```python
from build123d import *

# Parameters (mm, degrees)
SKETCH2_R          = 9.75
CUT_EXTRUDE1_DEPTH = 92.158049562


with BuildPart() as part:
    # Sketch1 → Revolve1 (revolve)
    with BuildSketch(Plane.XY, mode=Mode.PRIVATE) as revolve1_sk:
        Polygon((-17.25, 0), (-21.459646018, 0), (-23.940788684, 5.845205819), (-27.718503352, 5.845205819), (-30.199646018, 0), (-35, 0), (-35, 6.35), (-62.5, 6.35), (-62.5, 22.3), (-27, 22.3), (-27, 25), (-17.25, 25), align=None)
    revolve(revolve1_sk.sketch.rotate(Axis((0, 0, 0), (0, 1, 0)), 270), axis=Axis((0, 0, 0), (0, 1, 0)))

    # Sketch2 → Cut-Extrude1 (cut, through all)
    with BuildSketch(Plane(origin=(0, 22.3, 0), x_dir=(1, 0, 0), z_dir=(0, 1, 0))):
        with Locations(Location((-44.45, 0, 0), (0, 0, 270))):
            Circle(SKETCH2_R)
        with Locations(Location((0, 44.45, 0), (0, 0, 270))):
            Circle(SKETCH2_R)
        with Locations(Location((44.45, 0, 0), (0, 0, 270))):
            Circle(SKETCH2_R)
        with Locations(Location((0, -44.45, 0), (0, 0, 270))):
            Circle(SKETCH2_R)
    extrude(amount=-CUT_EXTRUDE1_DEPTH, mode=Mode.SUBTRACT)


solid = part.part
```
Work out the finished part from the listing and answer in its coordinate system (mm). A direction names the side the tool comes from. Give positions to 0.01 mm unless a question says otherwise; leave off trailing zeros. Order: outer loops, then holes, each group sorted by start corner. A loop starts at its lowest first (then second) coordinate and runs counter-clockwise, first axis right, second up. Notation, with made-up numbers: (63, 56.25) - (101, 56.25) arc R22 cw to (101, 63.25) - close; hole circle Ø4 at (88, -4). An arc over 180 degrees is marked (long way). One line per item, written item: value. Start each with the question number.
1. Section D-D, the plane z = -47 is taken. Write down the section's boundary in (x, y).
2. Section B-B, the plane z = 0 is taken. Write down the section's boundary in (x, y).
3. Which of the six approach directions +Z, -Z, +X, -X, +Y, -Y give full straight-line access (tool end or side, diameter ignored) to faces 1 (the face through (-24.999, 3.219, 24.496)), 2 (the face through (26.36, 23.67, 5.85)), 3 (the face through (12, 5.845, -21))?
4. Section C-C, the plane y = 11.25 is taken. Write down the section's boundary in (x, z).
5. Each of these flat-tipped pins is pushed along its axis until it touches: pin 1 Ø4 at (y, z) = (16.5, -49) entering from +X; pin 2 Ø6 at (y, z) = (9.5, 47) entering from +X; pin 3 Ø10 at (x, y) = (27.5, 17) entering from -Z. Where does it stop, or does it pass through?
6. Section A-A, the plane x = 0 is taken. Write down the section's boundary in (y, z).
7. For a pull along Z with two mould halves and no side action, classify faces 4 (the face through (0.43, 13.78, -54.19)), 5 (the face through (27, 6.35, 27)), 6 (the face through (-24.496, 3.219, -24.999)), 7 (the face through (-6.49, 0.37, -20.62)) as released by +Z, released by -Z, zero draft, split by the parting line, or undercut.
8. Consider line 1 (X direction, y = 8.5, z = 0); line 2 (X direction, y = 21, z = -3.5); line 3 (Z direction, x = 14, y = 5.75). Determine where each line is inside the solid, lowest interval first.
Filled sheet:
1. outline: (-41.2, 6.35) - (-9.41, 6.35) - (-9.41, 22.3) - (-41.2, 22.3) - close; (9.41, 6.35) - (41.2, 6.35) - (41.2, 22.3) - (9.41, 22.3) - close
2. outline: (-62.5, 6.35) - (-54.2, 6.35) - (-54.2, 22.3) - (-62.5, 22.3) - close; (-34.7, 0) - (-30.2, 0) - (-27.72, 5.85) - (-23.94, 5.85) - (-21.46, 0) - (-17.25, 0) - (-17.25, 25) - (-27, 25) - (-27, 22.3) - (-34.7, 22.3) - close; (17.25, 0) - (21.46, 0) - (23.94, 5.85) - (27.72, 5.85) - (30.2, 0) - (34.7, 0) - (34.7, 22.3) - (27, 22.3) - (27, 25) - (17.25, 25) - close; (54.2, 6.35) - (62.5, 6.35) - (62.5, 22.3) - (54.2, 22.3) - close
3. face 1: +Z, -X, -Y
3. face 2: +Y
3. face 3: -Y
4. outline: circle Ø125 at (0, 0); hole circle Ø19.5 at (-44.45, 0); hole circle Ø34.5 at (0, 0); hole circle Ø19.5 at (0, -44.45); hole circle Ø19.5 at (0, 44.45); hole circle Ø19.5 at (44.45, 0)
5. pin 1: x = 41.2
5. pin 2: x = 44.39
5. pin 3: z = -58.31
6. outline: (0, -34.7) - (22.3, -34.7) - (22.3, -27) - (25, -27) - (25, -17.25) - (0, -17.25) - (0, -21.46) - (5.85, -23.94) - (5.85, -27.72) - (0, -30.2) - close; (0, 17.25) - (25, 17.25) - (25, 27) - (22.3, 27) - (22.3, 34.7) - (0, 34.7) - (0, 30.2) - (5.85, 27.72) - (5.85, 23.94) - (0, 21.46) - close; (6.35, -62.5) - (22.3, -62.5) - (22.3, -54.2) - (6.35, -54.2) - close; (6.35, 54.2) - (22.3, 54.2) - (22.3, 62.5) - (6.35, 62.5) - close
7. face 4: undercut
7. face 5: zero draft
7. face 6: released by -Z
7. face 7: undercut
8. line 1: -62.5 to -54.2, -34.7 to -17.25, 17.25 to 34.7, 54.2 to 62.5
8. line 2: -62.4 to -53.55, -35.35 to -16.89, 16.89 to 35.35, 53.55 to 62.4
8. line 3: -32.08 to -23.97, -19.37 to -10.08, 10.08 to 19.37, 23.97 to 32.08
